Here's how the part is built. I have some questions about the finished solid (model axes, mm). A direction names the side the tool comes from. Coordinates: 2 decimals unless noted, no trailing zeros. Write each loop counter-clockwise with the first axis right and the second up, starting at its lowest first coordinate (ties: lowest second). Pieces come first, ordered by that corner, then holes. Notation, with made-up numbers: M -22.75,13 L 28.25,13 A18 cw 28.25,18 Z; hole C -7.5,18 d5. An arc over 180 degrees is marked long. Use a Markdown table: item, result.
```python
from build123d import *

# Parameters (mm, degrees)
BOSS_EXTRUDE2_DEPTH      = 7
CORTAR_REVOLUCI_N1_ANGLE = 180
REDONDEO1_START          = -5
REDONDEO1_DEPTH          = 10


with BuildPart() as part:
    # Sketch1 → Boss-Extrude2 (new, symmetric)
    with BuildSketch(Plane.XY):
        with BuildLine():
            Line((25.547749412, -14.75), (29.877876431, -17.25))
            ThreePointArc((29.877876431, -17.25), (33.324441007, -8.929257056), (34.5, 0))
            Line((34.5, 0), (34.5, 41.1))
            Line((34.5, 41.1), (31.075, 41.1))
            Line((31.075, 41.1), (31.075, 38.1))
            Line((31.075, 38.1), (-31.075, 38.1))
            Line((-31.075, 38.1), (-31.075, 41.1))
            Line((-31.075, 41.1), (-34.5, 41.1))
            Line((-34.5, 41.1), (-34.5, 0))
            ThreePointArc((-34.5, 0), (-33.324441007, -8.929257056), (-29.877876431, -17.25))
            Line((-29.877876431, -17.25), (-25.547749412, -14.75))
            ThreePointArc((-25.547749412, -14.75), (0, 29.5), (25.547749412, -14.75))
        make_face()
        with BuildLine():
            Line((-25, 34.925), (-19.25, 34.925))
            ThreePointArc((-19.25, 34.925), (-17.6625, 33.3375), (-19.25, 31.75))
            Line((-19.25, 31.75), (-25, 31.75))
            ThreePointArc((-25, 31.75), (-26.5875, 33.3375), (-25, 34.925))
        make_face(mode=Mode.SUBTRACT)
        with BuildLine():
            Line((19.25, 34.925), (25, 34.925))
            ThreePointArc((25, 34.925), (26.5875, 33.3375), (25, 31.75))
            Line((25, 31.75), (19.25, 31.75))
            ThreePointArc((19.25, 31.75), (17.6625, 33.3375), (19.25, 34.925))
        make_face(mode=Mode.SUBTRACT)
    extrude(amount=BOSS_EXTRUDE2_DEPTH, both=True)

    # Croquis1 → Cortar-Revolución1 (revolve, symmetric, cut)
    with BuildSketch(Plane(origin=(0, 0, 0), x_dir=(0, 0, -1), z_dir=(1, 0, 0))) as cortar_revoluci_n1_sk:
        with BuildLine():
            Line((-2.8575, 36.3375), (2.8575, 36.3375))
            ThreePointArc((2.8575, 36.3375), (4.445, 34.75), (2.8575, 33.1625))
            Line((2.8575, 33.1625), (-2.8575, 33.1625))
            ThreePointArc((-2.8575, 33.1625), (-4.445, 34.75), (-2.8575, 36.3375))
        make_face()
    revolve(axis=Axis((0, 0, 0), (0, 0, 1)), revolution_arc=CORTAR_REVOLUCI_N1_ANGLE / 2, mode=Mode.SUBTRACT)
    revolve(cortar_revoluci_n1_sk.sketch, axis=Axis((0, 0, 0), (0, 0, -1)), revolution_arc=CORTAR_REVOLUCI_N1_ANGLE / 2, mode=Mode.SUBTRACT)

    # Redondeo1: read off the stored shape, not the designer's step
    # Redondeo1 outline → Redondeo1 (add)
    with BuildSketch(Plane.XY.offset(REDONDEO1_START)):
        with BuildLine():
            ThreePointArc((34.5, 0), (33.514807302, 0.868494137), (33.095116255, 2.112980435))
            ThreePointArc((33.095116255, 2.112980435), (33.145649783, 1.057027304), (33.1625, 0))
            Line((33.1625, 0), (34.5, 0))
        make_face()
        with BuildLine():
            ThreePointArc((-33.095116255, 2.112980435), (-33.514807302, 0.868494137), (-34.5, 0))
            Line((-34.5, 0), (-33.1625, 0))
            ThreePointArc((-33.1625, 0), (-33.145649783, 1.057027304), (-33.095116255, 2.112980435))
        make_face()
    extrude(amount=REDONDEO1_DEPTH)


solid = part.part
```
1. Will these pins go through, and if not, where does the flat tip stop? pin 1 Ø6.5 at (x, z) = (23.5, -3) entering from +Y; pin 2 Ø3 at (x, z) = (23, -2.5) entering from -Y; pin 3 Ø8 at (y, z) = (-4, 4.5) entering from -X; pin 4 Ø6.5 at (x, z) = (-22.5, 2.5) entering from -Y.
Answers follow:
| item | result |
|---|---|
| pin 1 | stops at y = 38.1 |
| pin 2 | stops at y = 16.43 |
| pin 3 | stops at x = -34.5 |
| pin 4 | stops at y = -14.87 |
2. Suppose I cut it at A-A on z = 0.5. State how many separate pieces and enclosed holes the cut face has, and give its area (3 significant figures).
Answers follow:
| item | result |
|---|---|
| separate pieces | 2 |
| enclosed holes | 2 |
| area | 1,080 mm2 |
3. I need wall thicknesses on probe 1 along Y at (x, z) = (-22, 3) (3 decimals); probe 2 along X at (y, z) = (24, -2.5); probe 3 along Y at (x, z) = (23.5, -0.25) (3 decimals). Which ranges of each line are inside material? Lowest first, please.
Answers follow:
| item | result |
|---|---|
| probe 1 | y = 19.653 to 24.823, 28.913 to 31.75, 34.925 to 38.1 |
| probe 2 | x = -34.5 to -27.28, -22.89 to -17.15, 17.15 to 22.89, 27.28 to 34.5 |
| probe 3 | y = 17.833 to 23.399, 27.716 to 31.75, 34.925 to 38.1 |
4. We'd pull the mould along X, two halves only. Please class faces 1 (the face through (-22, 34.925, 0)), 2 (the face through (-5.3, 29.4, -7)), 3 (the face through (34.5, 25, 0)): +X half, -X half, draft (parallel to the pull), parting line (faces both ways), or undercut.
Answers follow:
| item | result |
|---|---|
| face 1 | undercut |
| face 2 | draft |
| face 3 | +X half |
5. Which directions (+Z, -Z, +X, -X, +Y, -Y) give clear straight access to the entire face, cutting with the end or side of a thin tool? Please do faces 4 (the face through (33.525, 0.853, -0.062)), 5 (the face through (31.075, 40, 0)), 6 (the face through (-22, 31.75, 0)), 7 (the face through (-27.743, -16.017, 0.098)), 8 (the face through (-0.7, 33.155, 0.04)).
Answers follow:
| item | result |
|---|---|
| face 4 | +X |
| face 5 | +Z, -Z, +Y |
| face 6 | +Z, -Z |
| face 7 | +Z, -Z, -Y |
| face 8 | none |
6. Suppose I cut it at C-C on y = -14. Write out the boundary of the cut face in (x, z).
Answers follow:
| item | result |
|---|---|
| outline | M -31.53,-7 L -25.97,-7 L -25.97,7 L -31.53,7 Z; M 25.97,-7 L 31.53,-7 L 31.53,7 L 25.97,7 Z |
